```python
from build123d import *

# Parameters (mm, degrees)
SKETCH1_R           = 1.75
SKETCH1_R_2         = 1
BOSS_EXTRUDE1_DEPTH = 2
SKETCH4_W           = 6
SKETCH4_H           = 6
BOSS_EXTRUDE2_DEPTH = 4
SKETCH5_R           = 2
CUT_EXTRUDE4_DEPTH  = 2


with BuildPart() as part:
    # Sketch1 → Boss-Extrude1 (new body)
    with BuildSketch(Plane.XY):
        with Locations((-39.967897534, 24.79140814)):
            Circle(SKETCH1_R)
        with Locations((-39.967897534, 24.79140814)):
            Circle(SKETCH1_R_2, mode=Mode.SUBTRACT)
    extrude(amount=BOSS_EXTRUDE1_DEPTH)

    # Sketch4 → Boss-Extrude2 (add)
    with BuildSketch(Plane.XY.offset(2)):
        with Locations((-39.967897534, 24.79140814)):
            Rectangle(SKETCH4_W, SKETCH4_H)
    extrude(amount=BOSS_EXTRUDE2_DEPTH)

    # Sketch5 → Cut-Extrude4 (cut)
    with BuildSketch(Plane.XY.offset(6)):
        with Locations((-39.967897534, 24.79140814)):
            Circle(SKETCH5_R)
        Polygon((-36.967897534, 25.818240491), (-36.967897534, 23.818240491), (-39.967897534, 23.818240491), (-42.967897534, 23.818240491), (-42.967897534, 25.818240491), (-39.967897534, 25.818240491), align=None)
        Polygon((-40.967897534, 24.79140814), (-40.967897534, 27.79140814), (-38.967897534, 27.79140814), (-38.967897534, 24.79140814), (-38.967897534, 21.79140814), (-40.967897534, 21.79140814), align=None)
    extrude(amount=-CUT_EXTRUDE4_DEPTH, mode=Mode.SUBTRACT)


solid = part.part
```
CAD build for the part. Positions are in the model's coordinates, mm. A direction names the side the tool comes from. Round coordinates to 2 decimals unless told otherwise and drop trailing zeros. Loops run counter-clockwise (first coordinate to the right, second up) from the corner with the lowest first, then second, coordinate; pieces in that order, holes last. Notation, with made-up numbers: (-1.5, -2) - (9.5, -2) arc R18 ccw to (9.5, 15) - close; hole circle Ø4 at (-18, 67). An arc over 180 degrees is marked (long way). Return JSON: item names as keys, results as strings. Group by question number.
Q1. Band-saw the part on D-D on x = -41.35. Give the cut face in (y, z).
Q2. Band-saw the part on A-A on z = 5.25. Give the cut face in (x, y), plus the area to 3 significant figures.
Q3. Band-saw the part on C-C on x = -42.2. Give the cut face in (y, z).
Q4. Flat gauge pins, fed straight in: pin 1 Ø3 at (y, z) = (26, 1) entering from +X; pin 2 Ø1.8 at (x, y) = (-40.5, 24) entering from +Z. Where does each tip first touch, or does it go through?
Q5. Band-saw the part on B-B on y = 27.2. Give the cut face in (x, z).
Q6. Drill centre lines: line 1 along X through (y, z) = (22.25, 5.65); line 2 along Y through (x, z) = (-42.4, 4.15); line 3 along X through (y, z) = (25.45, 1.4). Where is each one in solid material? Low to high. Write a range as [from, to].
Q7. Tool access for faces 1 (the face through (-38.968, 22, 5)), 2 (the face through (-38, 25.818, 5)), 3 (the face through (-41.3, 26.2, 2)): list every direction of +Z, -Z, +X, -X, +Y, -Y with a clear straight run to the whole face (end or side of a thin tool).
Q8. Two-plate mould, pull along Y, no slides. Class faces 4 (the face through (-40, 25, 2)), 5 (the face through (-40.968, 27, 5)), 6 (the face through (-38.3, 25.32, 0.99)), 7 (the face through (-40, 21.791, 3.5)): +Y half, -Y half, draft (parallel to the pull), parting line (faces both ways), or undercut.
Solutions:
{
 "1": {"outline": "(21.79, 2) - (23.72, 2) - (23.72, 0) - (25.86, 0) - (25.86, 2) - (27.79, 2) - (27.79, 6) - (26.24, 6) - (26.24, 4) - (23.35, 4) - (23.35, 6) - (21.79, 6) - close"},
 "2": {"outline": "(-42.97, 21.79) - (-40.97, 21.79) - (-40.97, 23.06) arc R2 cw to (-41.72, 23.82) - (-42.97, 23.82) - close; (-42.97, 25.82) - (-41.68, 25.82) arc R2 cw to (-40.97, 26.52) - (-40.97, 27.79) - (-42.97, 27.79) - close; (-38.97, 21.79) - (-36.97, 21.79) - (-36.97, 23.82) - (-38.22, 23.82) arc R2 cw to (-38.97, 23.06) - close; (-38.97, 26.52) arc R2 cw to (-38.25, 25.82) - (-36.97, 25.82) - (-36.97, 27.79) - (-38.97, 27.79) - close", "area": "14.7 mm^2"},
 "3": {"outline": "(21.79, 2) - (27.79, 2) - (27.79, 6) - (25.82, 6) - (25.82, 4) - (23.82, 4) - (23.82, 6) - (21.79, 6) - close"},
 "4": {"pin 1": "stops at x = -36.97", "pin 2": "stops at z = 4"},
 "5": {"outline": "(-42.97, 2) - (-36.97, 2) - (-36.97, 6) - (-38.97, 6) - (-38.97, 4) - (-40.97, 4) - (-40.97, 6) - (-42.97, 6) - close"},
 "6": {"line 1": "x = [-42.97, -40.97], [-38.97, -36.97]", "line 2": "y = [21.79, 23.82], [25.82, 27.79]", "line 3": "x = [-41.59, -40.72], [-39.22, -38.35]"},
 "7": {"face 1": "+Z, +Y, -Y", "face 2": "+Z, +X, -X", "face 3": "-Z"},
 "8": {"face 4": "undercut", "face 5": "draft", "face 6": "parting line", "face 7": "-Y half"}
}
